For this review, use the dimensioned drawing (mm, ordinates from the lowest corner) and the shaded views. A direction names the side the tool comes from. Coordinates: 2 decimals unless noted, no trailing zeros. Write each loop counter-clockwise with the first axis right and the second up, starting at its lowest first coordinate (ties: lowest second). Pieces come first, ordered by that corner, then holes. Notation, with made-up numbers: (65, 36.25) - (124, 36.25) arc R28 ccw to (124, 61.25) - close; hole circle Ø11 at (9.5, 83.25). An arc over 180 degrees is marked (long way). Answer as a JSON object with one key per item and string values.
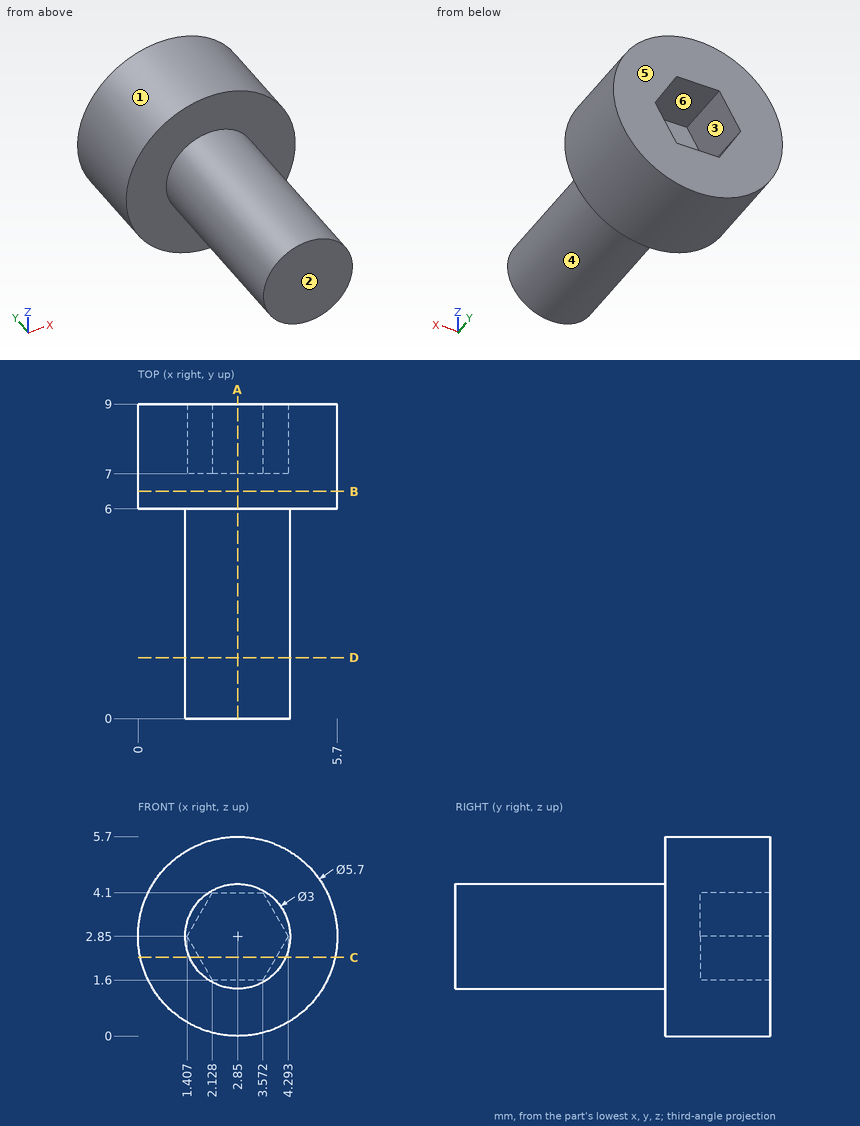
(1) For pin 1 (1 mm diameter, centred on y = 4, z = 2.5, fed in from +X); pin 2 (0.7 mm diameter, centred on x = 3, y = 8, fed in from +Z); pin 3 (1.5 mm diameter, centred on x = 4.5, y = 6.5, fed in from +Z); pin 4 (0.7 mm diameter, centred on x = 3.5, z = 2.5, fed in from +Y), all flat-tipped, find the tip position at first contact; note any pin that passes through.
Solved:
{"pin 1": "stops at x = 4.35", "pin 2": "stops at z = 5.7", "pin 3": "stops at z = 5.55", "pin 4": "stops at y = 7"}
(2) Tool access review of the marked faces 4, 5 and 6: name each direction out of +Z, -Z, +X, -X, +Y, -Y from which nothing blocks a thin tool from reaching the whole face with its end or side.
Solved:
{"face 4": "-Y", "face 5": "+Z, -Z, +X, -X, +Y", "face 6": "+Y"}
(3) Take a section at B-B, the plane y = 6.5. Write out the cut boundary in (x, z), and give its area (3 significant figures).
Solved:
{"outline": "circle Ø5.7 at (2.85, 2.85)", "area": "25.5 mm^2"}
(4) The part is to be moulded in two halves that separate along X. For the marked faces 1, 2 and 3, say which applies: pulls with the +X half, pulls with the -X half, needs draft (parallel to the pull), parting line crosses it, or undercut.
Solved:
{"face 1": "parting line crosses it", "face 2": "needs draft", "face 3": "undercut"}
(5) Take a section at D-D, the plane y = 1.75. Write out the cut boundary in (x, z).
Solved:
{"outline": "circle Ø3 at (2.85, 2.85)"}
(6) Take a section at C-C, the plane z = 2.25. Write out the cut boundary in (x, y) (1 decimal).
Solved:
{"outline": "(0.1, 6) - (1.5, 6) - (1.5, 0) - (4.2, 0) - (4.2, 6) - (5.6, 6) - (5.6, 9) - (3.9, 9) - (3.9, 7) - (1.8, 7) - (1.8, 9) - (0.1, 9) - close"}
(7) Take a section at A-A, the plane x = 2.85. Write out the cut boundary in (y, z).
Solved:
{"outline": "(0, 1.35) - (6, 1.35) - (6, 0) - (9, 0) - (9, 1.6) - (7, 1.6) - (7, 4.1) - (9, 4.1) - (9, 5.7) - (6, 5.7) - (6, 4.35) - (0, 4.35) - close"}
(8) To check wall thickness, follow line 1 (Y direction, x = 0.5, z = 2); line 2 (X direction, y = 5.5, z = 2.85); line 3 (Y direction, x = 3.85, z = 3.5). State the ranges of each line that lie inside material, in increasing order. Write a range as from..to.
Solved:
{"line 1": "y = 6..9", "line 2": "x = 1.35..4.35", "line 3": "y = 0..7"}
